from build123d import *

# Parameters (mm, degrees)
SKETCH1_R             = 40
TRUNK_DEPTH           = 580
BRANCH_BASE_PROFILE_R = 25
BRANCHES_COUNT        = 4


with BuildPart() as part:
    # Sketch1 → trunk (new body)
    with BuildSketch(Plane(origin=(0, 0, 0), x_dir=(1, 0, 0), z_dir=(0, 1, 0))):
        with Locations(Location((0, 0, 0), (0, 0, 270))):
            Circle(SKETCH1_R)
    extrude(amount=TRUNK_DEPTH)

    # branch base: sweep along a path in Sketch2
    with BuildLine(Plane(origin=(0, 0, 0), x_dir=(0, 0, -1), z_dir=(1, 0, 0))) as branch_base_path:
        Line((0, 600), (-450, 600))
    # branch base profile (on start of the path) → branch base (sweep)
    with BuildSketch(Plane(origin=(0, 600, 0), x_dir=(0, 1, 0), z_dir=(0, 0, 1))):
        Circle(BRANCH_BASE_PROFILE_R)
    branch_base = sweep(path=branch_base_path.line)

    # branches: branch base ×4 about axis
    branches_axis = Axis((0, 0, 0), (0, 1, 0))
    for i in range(1, BRANCHES_COUNT):
        add(branch_base.rotate(branches_axis, i * 360 / BRANCHES_COUNT))


solid = part.part
Model file for the job. Use its own axes, mm. A direction names the side the tool comes from. Give positions to 0.01 mm unless a question says otherwise; leave off trailing zeros. Write each loop counter-clockwise with the first axis right and the second up, starting at its lowest first coordinate (ties: lowest second). Pieces come first, ordered by that corner, then holes. Notation, with made-up numbers: M 48,3 L 57,3 A32 cw 57,36 Z; hole C -0.75,-38.75 d3. An arc over 180 degrees is marked long. One line per item, written item: value. Start each with the question number.
Q1. 3-axis set-ups, long thin cutter, end or side, ignore diameter. For faces 5 (the cylindrical face through (21.08, 613.44, 221.85)), 6 (the cylindrical face through (-39.05, 285.94, -8.67)), 7 (the flat face through (-450, 600, 0)): which of +Z, -Z, +X, -X, +Y, -Y reach the whole face in a straight line?
Q2. Probe probe 1 along X at (y, z) = (597, 331.5); probe 2 along Z at (x, y) = (35, 150.5); probe 3 along Z at (x, y) = (410.5, 586). List the from-to ranges inside material, lowest first. Write a range as [from, to].
Q3. Saw through at C-C, the plane x = -295.5. Write the cut outline in (y, z), plus the area to 3 significant figures.
Q4. Saw through at A-A, the plane y = 600. Write the cut outline in (x, z), plus the area to 3 significant figures.
Q5. Saw through at B-B, the plane z = 57. Write the cut outline in (x, y).
Q6. Drop flat-ended pins along their axis: pin 1 Ø17.5 at (x, z) = (28.5, -30) entering from +Y; pin 2 Ø12 at (x, z) = (23, -292) entering from +Y; pin 3 Ø6.5 at (x, z) = (27, 26) entering from +Y. Give the stop position or say it passes through.
Q7. Two-plate mould, pull along Y, no slides. Class faces 1 (the flat face through (24, 580, 23)), 2 (the flat face through (1, 0, -1)), 3 (the flat face through (0, 600, 450)), 4 (the flat face through (-23, 580, 23)): +Y half, -Y half, draft (parallel to the pull), parting line (faces both ways), or undercut.
Output values:
1. face 5: +Z
1. face 6: -Y
1. face 7: +Z, -Z, -X, +Y, -Y
2. probe 1: x = [-24.82, 24.82]
2. probe 2: z = [-19.36, 19.36]
2. probe 3: z = [-20.71, 20.71]
3. outline: C 600,0 d50
3. area: 1,960 mm²
4. outline: M -450,-25 L -25,-25 L -25,-450 L 25,-450 L 25,-25 L 450,-25 L 450,25 L 25,25 L 25,450 L -25,450 L -25,25 L -450,25 Z
4. area: 87,500 mm²
5. outline: C 0,600 d50
6. pin 1: stops at y = 615.33
6. pin 2: stops at y = 618.33
6. pin 3: stops at y = 610.37
7. face 1: undercut
7. face 2: -Y half
7. face 3: draft
7. face 4: undercut
